Part print with two shaded views. Sizes in mm from the minimum x, y, z corner. Coordinates: 2 decimals unless noted, no trailing zeros. Loops run counter-clockwise (first coordinate to the right, second up) from the corner with the lowest first, then second, coordinate; pieces in that order, holes last.
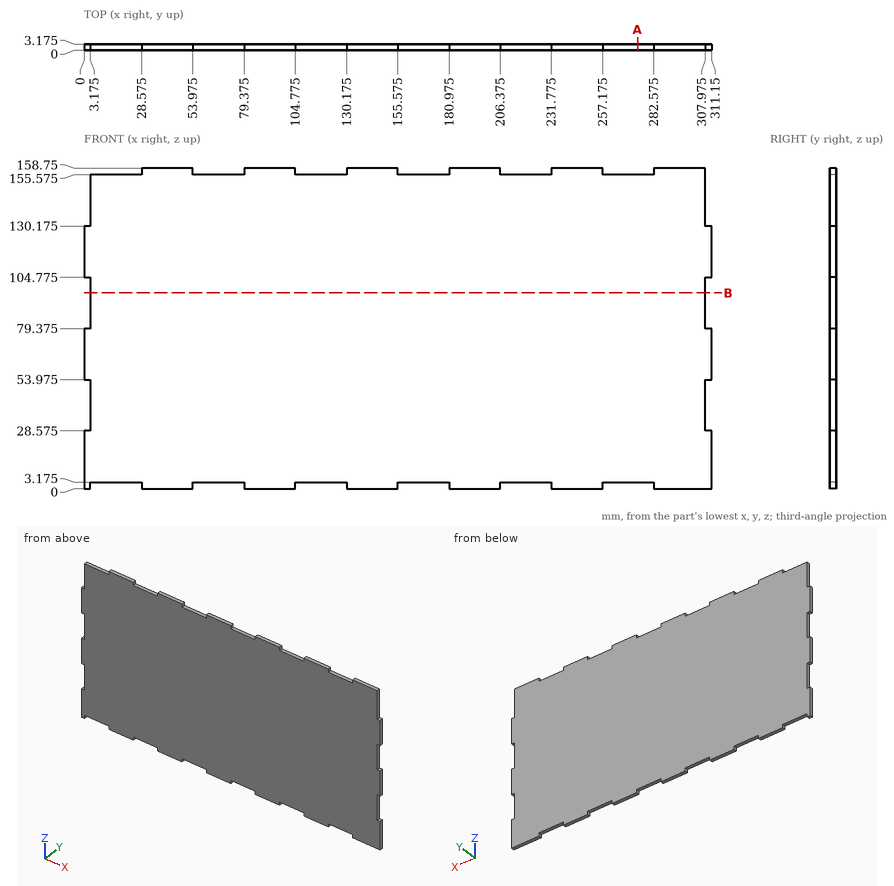
Q1. Slice it at A-A (x = 274.5). List the corners of the cut face in (y, z) (3 decimals), and give its area (3 significant figures).
Answers:
outline: (0, 3.175) - (3.175, 3.175) - (3.175, 155.575) - (0, 155.575) - close
area: 484 mm2
Q2. Flat gauge pins, fed straight in: P1, Ø1, axis at y = 1.5, z = 137.5, coming from the -X side (3 decimals); P2, Ø1.6, axis at x = 310, y = 1, coming from the +Z side (3 decimals); P3, Ø1.6, axis at x = 220, y = 1.5, coming from the -Z side (3 decimals). Where does each tip first touch, or does it go through?
Answers:
P1: stops at x = 3.175
P2: stops at z = 130.175
P3: stops at z = 3.175
Q3. Slice it at B-B (z = 97). List the corners of the cut face in (x, y) (3 decimals), and give its area (3 significant figures).
Answers:
outline: (3.175, 0) - (307.975, 0) - (307.975, 3.175) - (3.175, 3.175) - close
area: 968 mm2
Q4. Drill centre lines: line 1 (X direction, y = 0.75, z = 53) (3 decimals); line 2 (Z direction, x = 63, y = 1.85) (3 decimals). Where is each one in solid material? Low to high.
Answers:
line 1: x = 3.175 to 307.975
line 2: z = 3.175 to 155.575
